```python
from build123d import *

# Parameters (mm, degrees)
SKETCH2_W                      = 152.4
SKETCH2_H                      = 76.2
BOSS_EXTRUDE1_DEPTH            = 3.175
SKETCH3_W                      = 152.4
SKETCH3_H                      = 76.2
SKETCH3_W_2                    = 146.05
SKETCH3_H_2                    = 69.85
BOSS_EXTRUDE2_DEPTH            = 71.4375
SKETCH4_W                      = 152.4
SKETCH4_H                      = 76.2
BOSS_EXTRUDE3_DEPTH            = 3.175
SKETCH5_W                      = 152.4
SKETCH5_H                      = 76.2
SKETCH5_W_2                    = 146.05
SKETCH5_H_2                    = 69.85
BOSS_EXTRUDE4_DEPTH            = 98.425
F_97_1_DIAMETER_HOLE1_D        = 25.4
F_97_1_5_DIAMETER_HOLE1_D      = 38.1
F_97_1_5_DIAMETER_HOLE1_DEPTH  = 6.35
SKETCH6_W                      = 152.4
SKETCH6_H                      = 76.2
BOSS_EXTRUDE6_DEPTH            = 3.175
F_97_1_5_DIAMETER_HOLE2_D      = 38.1
F_97_1_5_DIAMETER_HOLE2_DEPTH  = 6.35
F_97_2_25_DIAMETER_HOLE1_D     = 57.15
F_97_2_25_DIAMETER_HOLE1_DEPTH = 6.35
SKETCH16_W                     = 152.4
SKETCH16_H                     = 76.2
SKETCH16_W_2                   = 146.05
SKETCH16_H_2                   = 69.85
BOSS_EXTRUDE7_DEPTH            = 23.8125
SKETCH17_W                     = 188.2
SKETCH17_H                     = 112.4
CUT_EXTRUDE1_DEPTH             = 3.175


with BuildPart() as part:
    # Sketch2 → Boss-Extrude1 (new body)
    with BuildSketch(Plane.YZ):
        with Locations((5.965836299, -2.847330961)):
            Rectangle(SKETCH2_W, SKETCH2_H)
    extrude(amount=BOSS_EXTRUDE1_DEPTH)

    # Sketch3 → Boss-Extrude2 (add)
    with BuildSketch(Plane.YZ.offset(3.175)):
        with Locations((5.965836299, -2.847330961)):
            Rectangle(SKETCH3_W, SKETCH3_H)
        with Locations((5.965836299, -2.847330961)):
            Rectangle(SKETCH3_W_2, SKETCH3_H_2, mode=Mode.SUBTRACT)
    extrude(amount=BOSS_EXTRUDE2_DEPTH)

    # Sketch4 → Boss-Extrude3 (add)
    with BuildSketch(Plane.YZ.offset(74.6125)):
        with Locations((5.965836299, -2.847330961)):
            Rectangle(SKETCH4_W, SKETCH4_H)
    extrude(amount=BOSS_EXTRUDE3_DEPTH)

    # Sketch5 → Boss-Extrude4 (add)
    with BuildSketch(Plane.YZ.offset(77.7875)):
        with Locations((5.965836299, -2.847330961)):
            Rectangle(SKETCH5_W, SKETCH5_H)
        with Locations((5.965836299, -2.847330961)):
            Rectangle(SKETCH5_W_2, SKETCH5_H_2, mode=Mode.SUBTRACT)
    extrude(amount=BOSS_EXTRUDE4_DEPTH)

    # #97 (1) Diameter Hole1 (through all)
    with Locations(Plane.YZ.offset(77.7875)):
        with Locations((-19.434163701, -2.847330961), (31.365836299, -2.847330961)):
            Hole(F_97_1_DIAMETER_HOLE1_D / 2)

    # #97 (1.5) Diameter Hole1
    with Locations(Plane(origin=(0, 0, 0), x_dir=(0, -1, 0), z_dir=(-1, 0, 0))):
        with Locations((-31.365836299, -2.847330961)):
            Hole(F_97_1_5_DIAMETER_HOLE1_D / 2, depth=F_97_1_5_DIAMETER_HOLE1_DEPTH)

    # Sketch6 → Boss-Extrude6 (add)
    with BuildSketch(Plane.YZ.offset(176.2125)):
        with Locations((5.965836299, -2.847330961)):
            Rectangle(SKETCH6_W, SKETCH6_H)
    extrude(amount=BOSS_EXTRUDE6_DEPTH)

    # #97 (1.5) Diameter Hole2
    with Locations(Plane.YZ.offset(179.3875)):
        with Locations((31.365836299, -2.847330961)):
            Hole(F_97_1_5_DIAMETER_HOLE2_D / 2, depth=F_97_1_5_DIAMETER_HOLE2_DEPTH)

    # #97 (2.25) Diameter Hole1
    with Locations(Plane.YZ.offset(179.3875)):
        with Locations((-19.434163701, -2.847330961)):
            Hole(F_97_2_25_DIAMETER_HOLE1_D / 2, depth=F_97_2_25_DIAMETER_HOLE1_DEPTH)

    # Sketch16 → Boss-Extrude7 (add)
    with BuildSketch(Plane.YZ.offset(179.3875)):
        with Locations((5.965836299, -2.847330961)):
            Rectangle(SKETCH16_W, SKETCH16_H)
        with Locations((5.965836299, -2.847330961)):
            Rectangle(SKETCH16_W_2, SKETCH16_H_2, mode=Mode.SUBTRACT)
    extrude(amount=BOSS_EXTRUDE7_DEPTH)

    # Sketch17 → Cut-Extrude1 (cut)
    with BuildSketch(Plane(origin=(0, 0, -40.947330961), x_dir=(1, 0, 0), z_dir=(0, 0, -1))):
        with Locations((109.1, -5.965836299)):
            Rectangle(SKETCH17_W, SKETCH17_H)
    extrude(amount=-CUT_EXTRUDE1_DEPTH, mode=Mode.SUBTRACT)


solid = part.part
```
The model under review builds one solid part; all positions refer to its coordinate system, in mm. A direction names the side the tool comes from. Round coordinates to 2 decimals unless told otherwise and drop trailing zeros. Write each loop counter-clockwise with the first axis right and the second up, starting at its lowest first coordinate (ties: lowest second). Pieces come first, ordered by that corner, then holes.
(1) Wall thickness on L1, parallel to X at y = -47.5, z = 14 (1 decimal); L2, parallel to Z at x = 11, y = 12; L3, parallel to Y at x = 92.5, z = 27: over which ranges is each line inside the solid? List them lowest first.
(2) Insertion check: pin 1 (12 mm diameter, centred on y = 26.5, z = -8.5, fed in from -X); pin 2 (5 mm diameter, centred on x = 32.5, y = -50, fed in from -Z); pin 3 (12 mm diameter, centred on x = 114, y = 22, fed in from -Z); pin 4 (3.5 mm diameter, centred on x = 177.5, y = -19.5, fed in from -Z). Each pin has a flat end and moves straight along its axis. Give the tip position at first contact, or say it passes through.
(3) We need section B-B on y = 31. Give the boundary of the cut face in (x, z) (1 decimal), and give its area (3 significant figures).
(4) We need section C-C on x = 86.5. Give the boundary of the cut face in (y, z).
(5) Machinability: for faces 1 (the flat face through (126, 5, 32.078)), 2 (the cylindrical face through (1.61, 49.536, 2.875)), 3 (the cylindrical face through (177.778, -15.714, 25.485)), which of the approach directions +Z, -Z, +X, -X, +Y, -Y give a long, thin tool a straight path to every point of the face, cutting with its end or side? Answer none if there is none.
(6) We need section D-D on z = -7.5. Give the number of separate pieces and of enclosed holes in the cut face, and give its area (3 significant figures).
(7) We need section A-A on y = -55.5. Give the boundary of the cut face in (x, z) (1 decimal).
(8) Mouldability with a two-part tool opening along X and no side actions: class faces 4 (the flat face through (179.388, 5, 13)), 5 (the flat face through (14.6, 4.9, -37.772)), 6 (the flat face through (100, 5, 35.253)) as +X half, -X half, draft (parallel to the pull), parting line (faces both ways), or undercut.
Findings below:
1. L1: x = 0 to 3.2, 74.6 to 77.8, 176.2 to 179.4
1. L2: z = -40.95 to -37.77, 32.08 to 35.25
1. L3: y = -70.23 to -67.06, 78.99 to 82.17
2. pin 1: stops at x = 74.61
2. pin 2: stops at z = -40.95
2. pin 3: stops at z = 32.08
2. pin 4: stops at z = -37.77
3. outline: (0, -40.9) - (15, -40.9) - (15, -37.8) - (3.2, -37.8) - (3.2, -21.9) - (0, -21.9) - close; (0, 16.2) - (3.2, 16.2) - (3.2, 32.1) - (74.6, 32.1) - (74.6, 9.8) - (77.8, 9.8) - (77.8, 32.1) - (176.2, 32.1) - (176.2, 16.2) - (179.4, 16.2) - (179.4, 32.1) - (203.2, 32.1) - (203.2, 35.3) - (0, 35.3) - close; (74.6, -37.8) - (77.8, -37.8) - (77.8, -15.5) - (74.6, -15.5) - close; (176.2, -37.8) - (179.4, -37.8) - (179.4, -21.9) - (176.2, -21.9) - close
3. area: 1,040 mm2
4. outline: (-70.23, -40.95) - (-50.23, -40.95) - (-50.23, -37.77) - (-67.06, -37.77) - (-67.06, 32.08) - (78.99, 32.08) - (78.99, -37.77) - (62.17, -37.77) - (62.17, -40.95) - (82.17, -40.95) - (82.17, 35.25) - (-70.23, 35.25) - close
5. face 1: none
5. face 2: -X
5. face 3: +X
6. separate pieces: 5
6. enclosed holes: 0
6. area: 2,040 mm2
7. outline: (0, -40.9) - (203.2, -40.9) - (203.2, -37.8) - (179.4, -37.8) - (179.4, 32.1) - (203.2, 32.1) - (203.2, 35.3) - (0, 35.3) - close; hole (3.2, -37.8) - (74.6, -37.8) - (74.6, 32.1) - (3.2, 32.1) - close; hole (77.8, -37.8) - (176.2, -37.8) - (176.2, 32.1) - (77.8, 32.1) - close
8. face 4: +X half
8. face 5: undercut
8. face 6: draft
